Build history of the part. All positions in model axes, mm. Face numbers are marked on the shaded views. Give positions to 0.01 mm unless a question says otherwise; leave off trailing zeros. Loops run counter-clockwise (first coordinate to the right, second up) from the corner with the lowest first, then second, coordinate; pieces in that order, holes last. Notation, with made-up numbers: M 82.5,-27.5 L 117.5,-27.5 A36 cw 117.5,10.5 Z; hole C -6.75,-30 d8. An arc over 180 degrees is marked long. Answer as a JSON object with one key per item and string values. Group by question number.
1. Slice it at B-B (z = -2.75). Give the number of separate pieces and of enclosed holes in the cut face, then the cut area to 3 significant figures.
2. Slice it at A-A (x = 0). List the corners of the cut face in (y, z), then the cut area to 3 significant figures.
3. Slice it at D-D (y = -1). List the corners of the cut face in (x, z).
4. Mould opens along Y. For the marked faces 1, 2 and 3 say: released by +Y, released by -Y, zero draft, split by the parting line, or undercut.
5. Drill centre lines: line 1 along Y through (x, z) = (0, -1.25); line 2 along Y through (x, z) = (2, 2); line 3 along X through (y, z) = (-3.5, 2.5). Where is each one in solid material? Low to high. Write a range as [from, to].
6. Drop flat-ended pins along their axis: pin 1 Ø2 at (x, z) = (23, -1) entering from -Y; pin 2 Ø4 at (x, y) = (0, 10) entering from -Z; pin 3 Ø1.5 at (y, z) = (6.5, -3.5) entering from +X; pin 4 Ø3 at (y, z) = (-4.5, -1.5) entering from +X. Give the stop position or say it passes through.
7. Slice it at C-C (x = 35). List the corners of the cut face in (y, z), then the cut area to 3 significant figures.
from build123d import *

# Parameters (mm, degrees)
ESQUISSE1_R        = 2.5
BOSS_EXTRU_1_DEPTH = 5
ESQUISSE2_R        = 5
BOSS_EXTRU_2_DEPTH = 46.6
CONG_1_R           = 3.883333333


with BuildPart() as part:
    # Esquisse1 → Boss.-Extru.1 (new, symmetric)
    with BuildSketch(Plane.XY):
        with BuildLine():
            Line((5, 10), (5, -10))
            ThreePointArc((5, -10), (0, -15), (-5, -10))
            Line((-5, -10), (-5, 10))
            ThreePointArc((-5, 10), (0, 15), (5, 10))
        make_face()
        with Locations((0, 10)):
            Circle(ESQUISSE1_R, mode=Mode.SUBTRACT)
        with Locations((0, -10)):
            Circle(ESQUISSE1_R, mode=Mode.SUBTRACT)
    extrude(amount=BOSS_EXTRU_1_DEPTH, both=True)

    # Esquisse2 → Boss.-Extru.2 (add)
    with BuildSketch(Plane(origin=(5, 0, 0), x_dir=(0, 0, -1), z_dir=(1, 0, 0))):
        with Locations((0, 5)):
            Circle(ESQUISSE2_R)
    extrude(amount=BOSS_EXTRU_2_DEPTH)

    # Congé1
    cong_1_edges = [part.edges().sort_by_distance(p)[0] for p in [
        (51.6, 5, 5),
    ]]
    fillet(cong_1_edges, radius=CONG_1_R)


solid = part.part
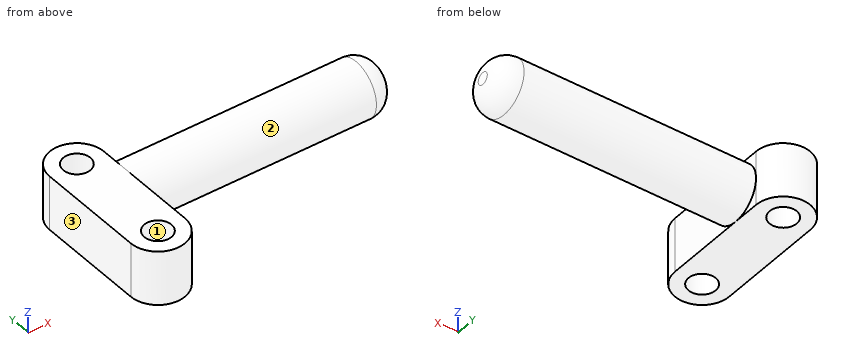
Established:
{
 "1": {"separate pieces": "1", "enclosed holes": "2", "area": "619 mm^2"},
 "2": {"outline": "M -15,-5 L -12.5,-5 L -12.5,5 L -15,5 Z; M -7.5,-5 L 7.5,-5 L 7.5,5 L -7.5,5 Z; M 12.5,-5 L 15,-5 L 15,5 L 12.5,5 Z", "area": "200 mm^2"},
 "3": {"outline": "M -5,-5 L 5,-5 L 5,5 L -5,5 Z"},
 "4": {"face 1": "undercut", "face 2": "split by the parting line", "face 3": "zero draft"},
 "5": {"line 1": "y = [-15, -12.5], [-7.5, 7.5], [12.5, 15]", "line 2": "y = [-14.58, -11.5], [-8.5, 8.5], [11.5, 14.58]", "line 3": "x = [-5, 5]"},
 "6": {"pin 1": "stops at y = 0", "pin 2": "passes through", "pin 3": "stops at x = 51.08", "pin 4": "stops at x = 5"},
 "7": {"outline": "C 5,0 d10", "area": "78.5 mm^2"}
}
